Part model, mm, in its own coordinate system. A direction names the side the tool comes from. Give positions to 0.01 mm unless a question says otherwise; leave off trailing zeros. Order: outer loops, then holes, each group sorted by start corner. A loop starts at its lowest first (then second) coordinate and runs counter-clockwise, first axis right, second up. Notation, with made-up numbers: (21.25, -19) - (69.25, -19) arc R25 cw to (69.25, 18) - close; hole circle Ø10 at (85, 2.5). An arc over 180 degrees is marked (long way). Use a Markdown table: item, result. Add a question column.
from build123d import *

# Parameters (mm, degrees)
F1_DEPTH = 138
F3_DEPTH = 49.4
F4_DEPTH = 78.6
F5_DEPTH = 25
F6_DEPTH = 25


with BuildPart() as f1:
    # F0 (on Front) → F1 (new body)
    with BuildSketch(Plane.XZ):
        with BuildLine():
            Line((-103.7269789477, -101.2127594065), (-100.3693379844, -95.8242133885))
            ThreePointArc((-100.3693379844, -95.8242133885), (-98.6798878596, -95.0745691606), (-98.2234282886, -96.8656171367))
            Line((-98.2234282886, -96.8656171367), (-132.6634080078, -153.5856345004))
            Line((-132.6634080078, -153.5856345004), (-143.4963060892, -171.4265906301))
            ThreePointArc((-143.4963060892, -171.4265906301), (-115.3707222455, -185.2538928172), (-104.207857368, -155.9685176268))
            Line((-104.207857368, -155.9685176268), (-105.7457237491, -156.770518844))
            ThreePointArc((-105.7457237491, -156.770518844), (-116.1787188571, -183.7071763743), (-141.9245898724, -170.6082820892))
            Line((-141.9245898724, -170.6082820892), (-97.3392441446, -97.179621432))
            ThreePointArc((-97.3392441446, -97.179621432), (-98.0067171309, -94.0759095516), (-101.1029781127, -94.7771338786))
            Line((-101.1029781127, -94.7771338786), (-115.8510804718, -118.4457837165))
            Line((-115.8510804718, -118.4457837165), (-120.663074613, -126.1683639899))
            Line((-120.663074613, -126.1683639899), (-119.7859828694, -126.7148860308))
            Line((-119.7859828694, -126.7148860308), (-114.8806803328, -119.0504468754))
            Line((-114.8806803328, -119.0504468754), (-108.5651855266, -108.950317898))
            Line((-108.5651855266, -108.950317898), (-103.7269789477, -101.2127594065))
        make_face()
    extrude(amount=F1_DEPTH)

    # F2 (on face) → F3 (cut)
    with BuildSketch(Plane(origin=(-28.0068430021, 0, 17.0055502417), x_dir=(0, 1, 0), z_dir=(0.8547686199, 0, -0.5190092546))):
        with BuildLine():
            Line((-41, -219.4907814326), (-41, -203.3049017191))
            ThreePointArc((-41, -203.3049017191), (-68.7405162983, -175.3061040983), (-96.9951905863, -202.7859566013))
            Line((-96.9951905863, -202.7859566013), (-96.9951905863, -203.8238468369))
            Line((-96.9951905863, -203.8238468369), (-96.9951905863, -219.4907814326))
            Line((-96.9951905863, -219.4907814326), (-41, -219.4907814326))
        make_face()
    extrude(amount=F3_DEPTH, mode=Mode.SUBTRACT)

    # F2 (on face) → F4 (cut)
    with BuildSketch(Plane(origin=(-28.0068430021, 0, 17.0055502417), x_dir=(0, 1, 0), z_dir=(0.8547686199, 0, -0.5190092546))):
        Polygon((-41, -251.147121191), (-41, -219.4907814326), (-96.9951905863, -219.4907814326), (-96.9951905863, -251.147121191), (-42.3506498337, -251.147121191), align=None)
    extrude(amount=F4_DEPTH, mode=Mode.SUBTRACT)

    # F2 (on face) → F5 (cut)
    with BuildSketch(Plane(origin=(-28.0068430021, 0, 17.0055502417), x_dir=(0, 1, 0), z_dir=(0.8547686199, 0, -0.5190092546))):
        with BuildLine():
            Line((-41, -219.4907814326), (-41, -203.3049017191))
            ThreePointArc((-41, -203.3049017191), (-68.7405162983, -175.3061040983), (-96.9951905863, -202.7859566013))
            Line((-96.9951905863, -202.7859566013), (-96.9951905863, -203.8238468369))
            Line((-96.9951905863, -203.8238468369), (-96.9951905863, -219.4907814326))
            Line((-96.9951905863, -219.4907814326), (-41, -219.4907814326))
        make_face()
    extrude(amount=-F5_DEPTH, mode=Mode.SUBTRACT)

    # F2 (on face) → F6 (cut)
    with BuildSketch(Plane(origin=(-28.0068430021, 0, 17.0055502417), x_dir=(0, 1, 0), z_dir=(0.8547686199, 0, -0.5190092546))):
        Polygon((-41, -251.147121191), (-41, -219.4907814326), (-96.9951905863, -219.4907814326), (-96.9951905863, -251.147121191), (-42.3506498337, -251.147121191), align=None)
    extrude(amount=-F6_DEPTH, mode=Mode.SUBTRACT)


solid = f1.part
1. Cut at A-A (y = -32). Write the cut outline in (x, z).
2. Cut at C-C (y = -66.5). Write the cut outline in (x, z).
3. Cut at B-B (x = -122.5). State how many separate pieces and enclosed holes the cut face has, plus the area to 3 significant figures.
4. Tool access for faces 5 (the face through (-117.37, -68.03, -122.94)), 6 (the face through (-126, 0, -143)), 7 (the face through (-103.008, -42.448, -164.905)): list every direction of +Z, -Z, +X, -X, +Y, -Y with a clear straight run to the whole face (end or side of a thin tool).
5. Mould opens along Z. For faces 1 (the face through (-115.83, -114.7, -185.43)), 2 (the face through (-128.9, -41, -184.4)), 3 (the face through (-103.22, -95.45, -164.42)), 4 (the face through (-102.1, -68, -98.6)) say: released by +Z, released by -Z, zero draft, split by the parting line, or undercut.
6. Drill centre lines: probe 1 along Z at (x, y) = (-103.5, -24.5); probe 2 along Z at (x, y) = (-113, -107); probe 3 along Z at (x, y) = (-118, -88). Where is each one in solid material? Low to high. Write a range as [from, to].
7. Pin check, flat tips, straight feed: P1, Ø1.5, axis at x = -99.21, z = -96.16, coming from the -Y side; P2, Ø3, axis at y = -118.5, z = -176, coming from the -X side; P3, Ø10, axis at y = -114.5, z = -132, coming from the +X side; P4, Ø6, axis at x = -105.5, y = -39, coming from the +Z side. Stop position of each tip, or through.
Responses:
| question | item | result |
|---|---|---|
| 1 | outline | (-143.5, -171.43) arc R21.2 ccw (long way) to (-104.21, -155.97) - (-105.75, -156.77) arc R19.47 cw (long way) to (-141.92, -170.61) - (-97.34, -97.18) arc R2.23 ccw (long way) to (-101.1, -94.78) - (-120.66, -126.17) - (-119.79, -126.71) - (-114.88, -119.05) - (-103.73, -101.21) - (-100.37, -95.82) arc R1.21 cw (long way) to (-98.22, -96.87) - close |
| 2 | outline | (-120.66, -126.17) - (-119.79, -126.71) - (-114.88, -119.05) - (-103.73, -101.21) - (-100.37, -95.82) arc R1.21 cw (long way) to (-98.22, -96.87) - (-119.84, -132.46) - (-119.05, -132.94) - (-97.34, -97.18) arc R2.23 ccw (long way) to (-101.1, -94.78) - close |
| 3 | separate pieces | 4 |
| 3 | enclosed holes | 0 |
| 3 | area | 325 mm² |
| 4 | face 5 | +Y, -Y |
| 4 | face 6 | +Z, -Z, +X, -X, +Y |
| 4 | face 7 | -Z, -X |
| 5 | face 1 | undercut |
| 5 | face 2 | zero draft |
| 5 | face 3 | released by -Z |
| 5 | face 4 | undercut |
| 6 | probe 1 | z = [-173.53, -157.52], [-107.33, -105.56], [-100.85, -98.62] |
| 6 | probe 2 | z = [-184.15, -182.15], [-122.97, -121.2], [-116.04, -113.87] |
| 6 | probe 3 | z = [-131.21, -129.44], [-123.92, -121.89] |
| 7 | P1 | passes through |
| 7 | P2 | stops at x = -142.34 |
| 7 | P3 | stops at x = -115.45 |
| 7 | P4 | stops at z = -97.02 |
